```python
from build123d import *

# Parameters (mm, degrees)
SKETCH1_R           = 10
SKETCH1_R_2         = 2.5
BOSS_EXTRUDE1_DEPTH = 6


with BuildPart() as part:
    # Sketch1 → Boss-Extrude1 (new body)
    # profile 1 of 3: a face of its own
    with BuildSketch(Plane(origin=(0, 0, 0), x_dir=(-1, 0, 0), z_dir=(0, 0, 1))):
        with Locations(Location((-8.506234752, 0, 0), (0, 0, 180))):
            Circle(SKETCH1_R)
        with Locations((-8.506234752, 0)):
            Circle(SKETCH1_R_2, mode=Mode.SUBTRACT)
    # profile 2 of 3: a face of its own
    with BuildSketch(Plane(origin=(0, 0, 0), x_dir=(-1, 0, 0), z_dir=(0, 0, 1))):
        with BuildLine():
            Line((-6.506234752, -1.5), (-10.506234752, -1.5))
            ThreePointArc((-10.506234752, -1.5), (-8.506234752, -2.5), (-6.506234752, -1.5))
        make_face()
    # profile 3 of 3: a face of its own
    with BuildSketch(Plane(origin=(0, 0, 0), x_dir=(-1, 0, 0), z_dir=(0, 0, 1))):
        with BuildLine():
            ThreePointArc((-6.506234752, 1.5), (-8.506234752, 2.5), (-10.506234752, 1.5))
            Line((-10.506234752, 1.5), (-6.506234752, 1.5))
        make_face()
    extrude(amount=BOSS_EXTRUDE1_DEPTH)


solid = part.part
```
Input: part model. Units: mm. Frame: model coordinates. A direction names the side the tool comes from. Coordinates: 2 decimals unless noted, no trailing zeros. Loops run counter-clockwise (first coordinate to the right, second up) from the corner with the lowest first, then second, coordinate; pieces in that order, holes last. Notation, with made-up numbers: M 36,4.25 L 72,4.25 A37 cw 72,42.25 Z; hole C 2,71.5 d11. An arc over 180 degrees is marked long. One line per item, written item: value.
(1) Section B-B (z = 3.5). Output: boundary loops of the cut face in (x, y), and give its area (3 significant figures).
Filled in:
outline: C 8.51,0 d20; hole M 6.51,-1.5 L 10.51,-1.5 A2.5 ccw 10.51,1.5 L 6.51,1.5 A2.5 ccw Z
area: 300 mm^2
(2) Pin query (flat end, axial travel): pin 1 (1.5 mm diameter, centred on x = 10.5, z = 2, fed in from -Y). Return the tip coordinate at first contact, or that it passes through.
Filled in:
pin 1: y = -9.92
(3) Section D-D (x = 0.5). Output: boundary loops of the cut face in (y, z), and give its area (3 significant figures).
Filled in:
outline: M -5.99,0 L 5.99,0 L 5.99,6 L -5.99,6 Z
area: 71.9 mm^2
(4) Pull-direction query (Y, two-part tool) for faces 1 (the flat face through (9, -1.5, 3)), 2 (the cylindrical face through (17.744, -3.83, 2.958)), 3 (the flat face through (8, -2, 0)); classes: +Y half, -Y half, draft (parallel to the pull), parting line (faces both ways), or undercut.
Filled in:
face 1: undercut
face 2: parting line
face 3: draft
(5) Reachability of faces 4 (the flat face through (8, -2, 6)), 5 (the flat face through (8, 1.5, 3)) from +Z, -Z, +X, -X, +Y, -Y: full face, straight path, thin tool, end or side. Return the list, or none.
Filled in:
face 4: +Z, +X, -X, +Y, -Y
face 5: +Z, -Z
(6) Line query: line 1 along Y through (x, z) = (7.5, 3.95); line 2 along Y through (x, z) = (10.25, 2.4); line 3 along X through (y, z) = (-0.75, 3.45). Output: solid intervals per line, ascending. Write a range as from..to.
Filled in:
line 1: -9.95..-1.5, 1.5..9.95
line 2: -9.85..-1.5, 1.5..9.85
line 3: -1.47..6.12, 10.89..18.48
(7) Section C-C (y = 4). Output: boundary loops of the cut face in (x, z), and give its area (3 significant figures).
Filled in:
outline: M -0.66,0 L 17.67,0 L 17.67,6 L -0.66,6 Z
area: 110 mm^2
(8) Section A-A (y = 0). Output: boundary loops of the cut face in (x, z), and give its area (3 significant figures).
Filled in:
outline: M -1.49,0 L 6.01,0 L 6.01,6 L -1.49,6 Z; M 11.01,0 L 18.51,0 L 18.51,6 L 11.01,6 Z
area: 90.0 mm^2
